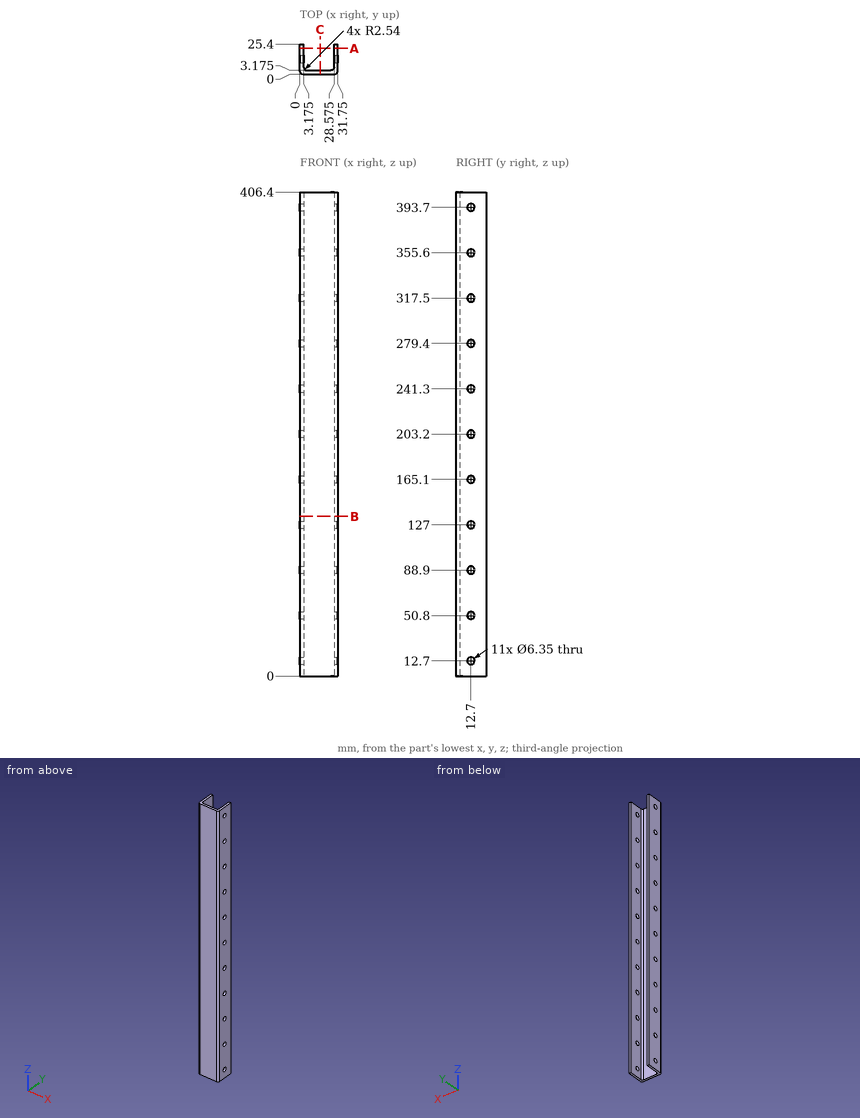
Verification items for this drawing (mm, ordinates from the low corner). Coordinates: 2 decimals unless noted, no trailing zeros. Order: outer loops, then holes, each group sorted by start corner. A loop starts at its lowest first (then second) coordinate and runs counter-clockwise, first axis right, second up. Notation, with made-up numbers: M 65.25,40.25 L 122.25,40.25 A17 ccw 122.25,53.25 Z; hole C 29,-25.75 d8. An arc over 180 degrees is marked long. Write each question's results on one line, items separated by ' | '.
1) Gauge pin test, flat end, axial feed: pin 1 Ø4 at (y, z) = (5, 218) entering from -X. Record the tip position at first contact, or that the pin passes through.
Solved:
pin 1: stops at x = 0
2) Section check C-C on x = 17. Record the cut outline in (y, z) (3 decimals).
Solved:
outline: M 0,0 L 3.175,0 L 3.175,406.4 L 0,406.4 Z
3) Section check B-B on z = 134. Record the cut outline in (x, y) (3 decimals), plus the area to 3 significant figures.
Solved:
outline: M 0,2.54 A2.54 ccw 2.54,0 L 29.21,0 A2.54 ccw 31.75,2.54 L 31.75,25.4 L 28.575,25.4 L 28.575,5.715 A2.54 cw 26.035,3.175 L 5.715,3.175 A2.54 cw 3.175,5.715 L 3.175,25.4 L 0,25.4 Z | area: 242 mm²
4) Scan lines: line 1 along Y through (x, z) = (2, 165.1) (3 decimals); line 2 along X through (y, z) = (19.75, 267.5) (3 decimals); line 3 along Y through (x, z) = (25, 80.5) (3 decimals). Record each from-to range of solid material in increasing order. Write a range as [from, to].
Solved:
line 1: y = [0.058, 9.525], [15.875, 25.4] | line 2: x = [0, 3.175], [28.575, 31.75] | line 3: y = [0, 3.175]
5) Section check A-A on y = 21.75. Record the cut outline in (x, z) (3 decimals), plus the area to 3 significant figures.
Solved:
outline: M 0,0 L 3.175,0 L 3.175,406.4 L 0,406.4 Z; M 28.575,0 L 31.75,0 L 31.75,406.4 L 28.575,406.4 Z | area: 2,580 mm²
